Geometry check sheet. Reference: the model listing, model coordinates, mm. Face numbers are marked on the shaded views. Round coordinates to 2 decimals unless told otherwise and drop trailing zeros. Order: outer loops, then holes, each group sorted by start corner. A loop starts at its lowest first (then second) coordinate and runs counter-clockwise, first axis right, second up.
(1) Sectioned sample at B-B (x = 0). Record the boundary of the cut face in (y, z), plus the area to 3 significant figures.
(2) Sectioned sample at D-D (y = 40). Record the boundary of the cut face in (x, z).
(3) Go/stop test with flat-tipped pins: pin 1 (7 mm diameter, centred on x = -15, y = 46, fed in from -Z); pin 2 (5 mm diameter, centred on x = -7, y = 12.12, fed in from -Z); pin 3 (6 mm diameter, centred on x = 16, y = 35.15, fed in from -Z); pin 4 (1.9 mm diameter, centred on x = -16, y = 35, fed in from -Z). Record where each tip stops, or that it passes through.
(4) Sectioned sample at A-A (y = -45.15). Record the boundary of the cut face in (x, z).
(5) Release check for a two-part mould opening along Z. For the marked faces 1, 2 and 3 record: +Z half, -Z half, draft (parallel to the pull), parting line (faces both ways), or undercut.
(6) Sectioned sample at C-C (z = 11.5). Give the number of separate pieces and of enclosed holes in the cut face, plus the area to 3 significant figures.
(7) Material ranges on line 1 along Y through (x, z) = (-16, 6.2); line 2 along X through (y, z) = (0, 10.7); line 3 along Y through (x, z) = (-16, 9.3), recorded low to high.
Autodesk Inventor part; units mm, degrees
ref_plane "YZ Plane" through (0, 0, 0) normal (1, 0, 0) x (0, 1, 0)
ref_plane "XZ Plane" through (0, 0, 0) normal (0, 1, 0) x (-1, 0, 0)
ref_plane "XY Plane" through (0, 0, 0) normal (0, 0, 1) x (1, 0, 0)
sketch "Sketch1" plane through (0, 0, 0) normal (0, 0, 1) x (1, 0, 0)
  circle A0 centre (0, 0) radius 17.5
  dimension "d0" = 35
extrude "Extrusion1" add sketch "Sketch1" along normal blind 5
sketch "Sketch2" plane through (0, 0, 5) normal (0, 0, 1) x (1, 0, 0)
  line L0 (-19, -50) -> (19, -50)
  line L1 (19, -50) -> (19, 50)
  line L2 (19, 50) -> (-19, 50)
  line L3 (-19, 50) -> (-19, -50)
  line L4 (-19, -50) -> (19, 50) construction
  line L5 (19, -50) -> (-19, 50) construction
  point P0 (0, 0)
  dimension "d3" = 38
  dimension "d4" = 100
extrude "Extrusion2" add sketch "Sketch2" along normal blind 8
sketch "Sketch3" plane through (0, 0, 13) normal (0, 0, 1) x (1, 0, 0)
  point P0 (0, 0)
  point P1 (14, 0)
  dimension "d7" = 14
hole "Hole1" at (14, 0, 13) direction (0, 0, -1) diameter 3.4 end through all counterbore diameter 6.5 counterbore depth 4
pattern_circular "Circular Pattern1" count 6 over 360 about axis through (0, 0, -10) along (0, 0, 1) of "Hole1"
sketch "Sketch4" plane through (0, 0, 5) normal (0, 0, -1) x (-1, 0, 0)
  line L0 (-16, 45.15) -> (16, 45.15)
  line L1 (16, 45.15) -> (16, 35.15)
  line L2 (16, 35.15) -> (-16, 35.15)
  line L3 (-16, 35.15) -> (-16, 45.15)
  line L4 (-16, 45.15) -> (16, 35.15) construction
  line L5 (16, 45.15) -> (-16, 35.15) construction
  line L6 (-19, 50) -> (19, 50)
  line L7 (19, 50) -> (19, -50)
  line L8 (-19, -50) -> (-19, 50)
  point P0 (0, 0)
  point P1 (0, 40.15)
  dimension "d18" = 4.85
  dimension "d19" = 3
  dimension "d20" = 3
  dimension "d21" = 10
hole "Hole2" at (16, 45.15, 5) at (-16, 45.15, 5) at (-16, 35.15, 5) at (16, 35.15, 5) direction (0, 0, 1) diameter 3.4 end through all counterbore diameter 6.5 counterbore depth 3.4
mirror "Mirror1" about plane through (0, 0, 0) normal (0, 1, 0) of "Hole2"
fillet "Fillet1" radius 2 1 edges at (-17.5, 0, 5)
ref_plane "Work Plane1" through (0, 0, 0) normal (0, 1, 0) x (-1, 0, 0)
equation "\"d19\" = d20"
properties part number "401-flange"
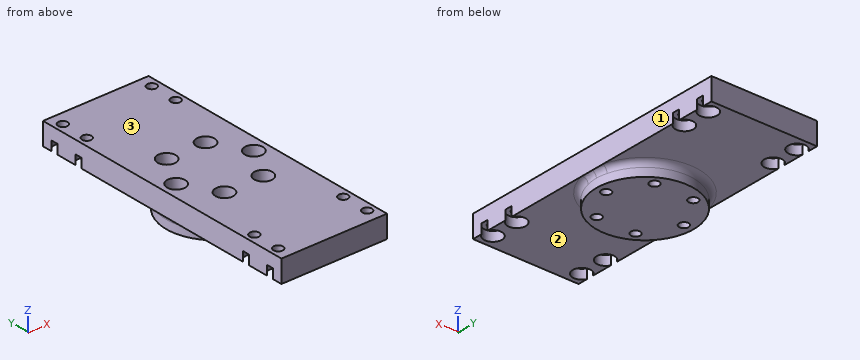
Answer below:
1. outline: (-50, 5) - (-19.5, 5) arc R2 cw to (-17.5, 3) - (-17.5, 0) - (17.5, 0) - (17.5, 3) arc R2 cw to (19.5, 5) - (50, 5) - (50, 13) - (-50, 13) - close
1. area: 977 mm2
2. outline: (-19, 5) - (19, 5) - (19, 13) - (-19, 13) - close
3. pin 1: stops at z = 5
3. pin 2: stops at z = 0
3. pin 3: stops at z = 8.4
3. pin 4: passes through
4. outline: (-19, 8.4) - (-17.7, 8.4) - (-17.7, 13) - (-19, 13) - close; (-14.3, 8.4) - (-12.75, 8.4) - (-12.75, 5) - (12.75, 5) - (12.75, 8.4) - (14.3, 8.4) - (14.3, 13) - (-14.3, 13) - close; (17.7, 8.4) - (19, 8.4) - (19, 13) - (17.7, 13) - close
5. face 1: draft
5. face 2: -Z half
5. face 3: +Z half
6. separate pieces: 1
6. enclosed holes: 14
6. area: 3,530 mm2
7. line 1: y = -50 to -48.4, -41.9 to -38.4, -31.9 to 31.9, 38.4 to 41.9, 48.4 to 50
7. line 2: x = -19 to -17.25, -10.75 to 10.75, 17.25 to 19
7. line 3: y = -50 to -46.85, -43.45 to -36.85, -33.45 to -2.56, 2.56 to 33.45, 36.85 to 43.45, 46.85 to 50
